Drawing for the job (mm, zero at the part's lowest x, y, z). Give positions to 0.01 mm unless a question says otherwise; leave off trailing zeros. Loops run counter-clockwise (first coordinate to the right, second up) from the corner with the lowest first, then second, coordinate; pieces in that order, holes last. Notation, with made-up numbers: M 87.25,-18.75 L 102.25,-18.75 A8 ccw 102.25,-6.75 Z; hole C 84,-38 d10. An arc over 180 degrees is marked long. Use CSV: the item, a comma, the result in double quotes. Start each with the question number.
(1) Wall check: line 1 along Z through (x, y) = (5.75, 2.5); line 2 along X through (y, z) = (3.75, 3.95); line 3 along Y through (x, z) = (2.5, 0.25) (1 decimal). Give the ranges that are in metal, low to high. Write a range as from..to.
(2) Slice it at B-B on y = 4. List the corners of the cut face in (x, z).
(3) Slice it at A-A on x = 4. List the corners of the cut face in (y, z) (1 decimal).
(4) Two-plate mould, pull along X, no slides. Class the marked faces 1, 2, 3 and 4: pulls with the +X half, pulls with the -X half, needs draft (parallel to the pull), parting line crosses it, or undercut.
(5) Slice it at D-D on z = 3.6. List the corners of the cut face in (x, y).
(6) Flat gauge pin, fed straight in: P1, Ø3, axis at x = 2, y = 4, coming from the -Z side. Where does the tip first touch, or does it go through?
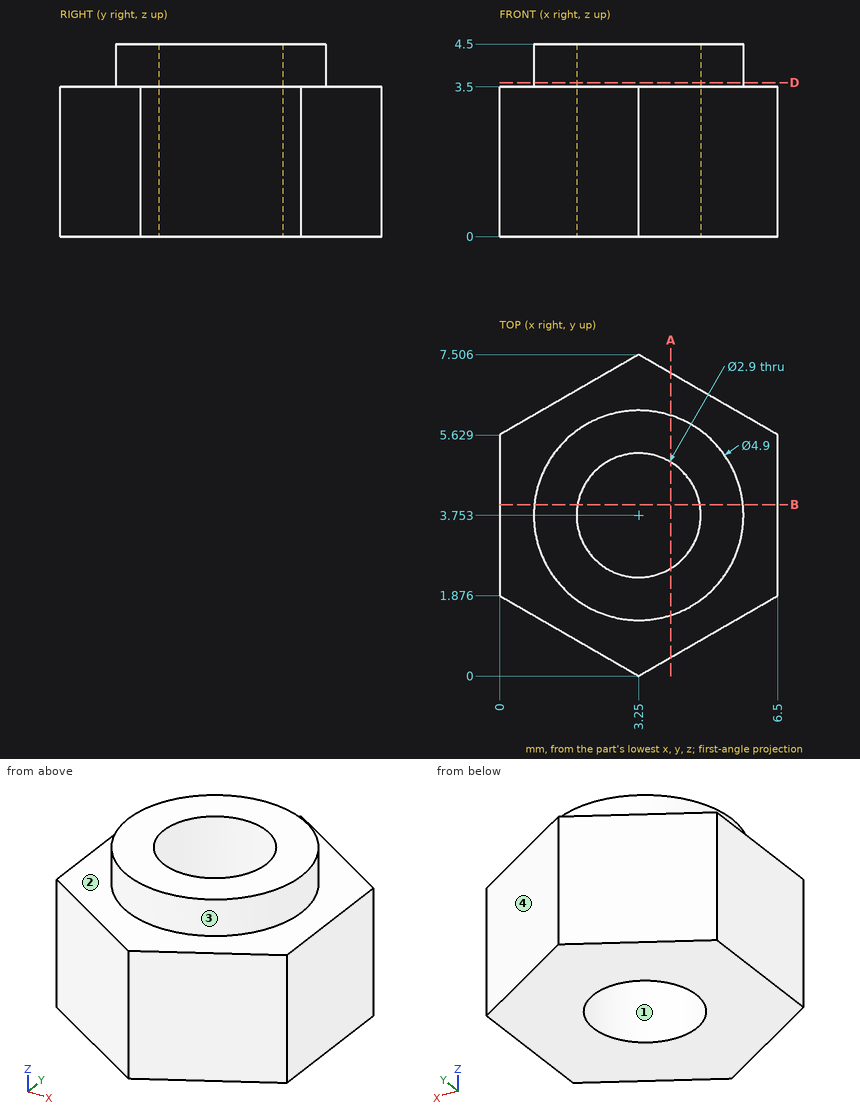
Reply:
1,line 1,"z = 0..3.5"
1,line 2,"x = 0.8..1.8, 4.7..5.7"
1,line 3,"y = 0.4..2.5, 5..7.1"
2,outline,"M 0,0 L 1.82,0 L 1.82,4.5 L 0.81,4.5 L 0.81,3.5 L 0,3.5 Z; M 4.68,0 L 6.5,0 L 6.5,3.5 L 5.69,3.5 L 5.69,4.5 L 4.68,4.5 Z"
3,outline,"M 0.4,0 L 2.5,0 L 2.5,4.5 L 1.4,4.5 L 1.4,3.5 L 0.4,3.5 Z; M 5,0 L 7.1,0 L 7.1,3.5 L 6.1,3.5 L 6.1,4.5 L 5,4.5 Z"
4,face 1,"undercut"
4,face 2,"needs draft"
4,face 3,"parting line crosses it"
4,face 4,"pulls with the +X half"
5,outline,"C 3.25,3.75 d4.9; hole C 3.25,3.75 d2.9"
6,P1,"stops at z = 0"
